```python
from build123d import *

# Parameters (mm, degrees)
F0_W      = 25.4
F0_H      = 50.8
F0_R      = 3.175
F0_R_2    = 6.35
F0_R_3    = 2.54
F1_DEPTH  = 6.35
F2_DEPTH  = 63.5
F4_DEPTH  = 6.35
F2_FACE_R = 6.35
F6_R      = 3.175


with BuildPart() as f1:
    # F0 (on Top) → F1 (new body)
    with BuildSketch(Plane.XY):
        Rectangle(F0_W, F0_H)
        with Locations((0, -19.2597191781)):
            Circle(F0_R, mode=Mode.SUBTRACT)
        Circle(F0_R_2, mode=Mode.SUBTRACT)
        with Locations((0, 18.014030531)):
            Circle(F0_R_3, mode=Mode.SUBTRACT)
    extrude(amount=F1_DEPTH)

    # F0 (on Top) → F2 (join)
    with BuildSketch(Plane.XY):
        Circle(F0_R_2)
    extrude(amount=F2_DEPTH)

    # F0 (on Top) → F4 (join, through all)
    with BuildSketch(Plane.XY):
        with Locations((0, -19.2597191781)):
            Circle(F0_R)
    extrude(amount=F4_DEPTH)

    # F5: sweep along a path in F3
    with BuildLine(Plane.YZ) as f5_path:
        add(Plane.YZ * Edge.make_bspline(
            [(0, 63.5), (0.3497077138, 64.9335091592), (1.0344697619, 70.7236922928), (8.5873221979, 75.9309157729), (13.3415265009, 77.8324604034)],
            knots=[0, 0, 0, 0, 0.400987996, 1, 1, 1, 1], degree=3))
    # F2_face (on face) → F5 (sweep)
    with BuildSketch(Plane.XY.offset(63.5)):
        Circle(F2_FACE_R)
    sweep(path=f5_path.line)

    # F7: sweep along a path in F3
    with BuildLine(Plane.YZ) as f7_path:
        Line((-19.2597191781, 6.35), (-6.35, 25.267848745))
    # F6 (on face) → F7 (sweep)
    with BuildSketch(Plane.XY.offset(6.35)):
        with Locations((0, -19.2597191781)):
            Circle(F6_R)
    sweep(path=f7_path.line)


solid = f1.part
```
Could you check a few things on this model? Use its own coordinates, in mm. A direction names the side the tool comes from. Round coordinates to 2 decimals unless told otherwise and drop trailing zeros. Write each loop counter-clockwise with the first axis right and the second up, starting at its lowest first coordinate (ties: lowest second). Pieces come first, ordered by that corner, then holes.
(1) Which directions (+Z, -Z, +X, -X, +Y, -Y) give clear straight access to the entire face, cutting with the end or side of a thin tool? Please do faces 1 (the face through (0, 25.4, 3)), 2 (the face through (3, 6, 6.35)).
Findings below:
face 1: +Z, -Z, +X, -X, +Y
face 2: none
(2) Suppose I cut it at A-A on z = 26.5. Write out the boundary of the cut face in (x, y).
Findings below:
outline: circle Ø12.7 at (0, 0)
(3) If I drill on probe 1 along Y at (x, z) = (0, 1.5); probe 2 along Z at (x, y) = (9.5, 13); probe 3 along Z at (x, y) = (-1.5, -14), over which ranges is the centre line in solid material (lowest first)?
Findings below:
probe 1: y = -25.4 to 15.47, 20.55 to 25.4
probe 2: z = 0 to 6.35
probe 3: z = 0 to 6.35, 9.96 to 18.16
(4) Thinking about a two-plate mould opening in Y: for faces 3 (the face through (0, -8, 25.268)), 4 (the face through (0, -25.4, 3)), 5 (the face through (-0.551, 15.534, 3.131)), which applies, +Y half, -Y half, draft (parallel to the pull), parting line (faces both ways), or undercut?
Findings below:
face 3: draft
face 4: -Y half
face 5: undercut
(5) Suppose I cut it at B-B on x = 0. State how many separate pieces and enclosed holes the cut face has, and give its area (3 significant figures).
Findings below:
separate pieces: 2
enclosed holes: 1
area: 1,380 mm2
(6) For pin 1 (12 mm diameter, centred on y = 19, z = 14, fed in from +X); pin 2 (2 mm diameter, centred on y = 5, z = 63.5, fed in from +X); pin 3 (6 mm diameter, centred on x = -8, z = 42.5, fed in from +Y); pin 4 (6 mm diameter, centred on y = 13.5, z = 71, fed in from +X), each with a flat end and sliding along its axis, tell me the tip position at first contact or that it passes through.
Findings below:
pin 1: passes through
pin 2: stops at x = 4.94
pin 3: stops at y = 3.91
pin 4: stops at x = 5.36
